Part model, mm, in its own coordinate system. A direction names the side the tool comes from. Round coordinates to 2 decimals unless told otherwise and drop trailing zeros. Write each loop counter-clockwise with the first axis right and the second up, starting at its lowest first coordinate (ties: lowest second). Pieces come first, ordered by that corner, then holes.
1) Flat gauge pins, fed straight in: pin 1 (12 mm diameter, centred on y = 2, z = 15, fed in from -X); pin 2 (15 mm diameter, centred on y = -8.5, z = -2, fed in from +X); pin 3 (21 mm diameter, centred on y = 9, z = -3, fed in from -X). Where does each tip first touch, or does it go through?
2) Drill centre lines: L1, parallel to X at y = 24, z = -9.5; L2, parallel to Z at x = 51, y = -9.5 (3 decimals); L3, parallel to Z at x = -148, y = -8 (3 decimals). Where is each one in solid material? Low to high.
3) Which spindle directions (+Z, -Z, +X, -X, +Y, -Y) get a long thin tool onto all of the face, cutting with end or side? Do faces 1 (the cylindrical face through (116.458, -0.533, 13.965)), 2 (the flat face through (127.794, -1, 0)), 3 (the flat face through (-14, -38.1, 17)). Say none if no direction does.
4) Saw through at B-B on z = -19. Write the cut outline in (x, y) (1 decimal), and give its area (3 significant figures).
5) Saw through at D-D on y = 0. Count the separate pieces of the cut face and the enclosed holes in it, and give its area (3 significant figures).
6) Saw through at A-A on z = 5. Write the cut outline in (x, y), and give its area (3 significant figures).
7) Pull direction X, two halves, no side cores. Call faces 4 (the cylindrical face through (123.02, -0.533, 20.873)), 5 (the flat face through (118.269, -1, 0)), 6 (the flat face through (-14, 38.1, 17)): +X half, -X half, draft (parallel to the pull), parting line (faces both ways), or undercut.
8) Saw through at C-C on y = 29. Write the cut outline in (x, z) (3 decimals), and give its area (3 significant figures).
```python
from build123d import *

# Parameters (mm, degrees)
F1_DEPTH = 38.1
F2_R     = 6.35
F3_R     = 15.875
F4_R     = 8.73125
F5_DEPTH = 25.4
F6_R     = 7.14375
F7_DEPTH = 25.4


with BuildPart() as f1:
    # F0 (on Front) → F1 (new body, symmetric)
    with BuildSketch(Plane.XZ):
        Polygon((-178.59375, -15.875), (-178.59375, -25.4), (-118.26875, -25.4), (-118.26875, 15.875), (118.26875, 15.875), (118.26875, -25.4), (178.59375, -25.4), (178.59375, -15.875), (127.79375, -15.875), (127.79375, 25.4), (-127.79375, 25.4), (-127.79375, -15.875), align=None)
    extrude(amount=F1_DEPTH, both=True)

    # F2
    f2_edges = [f1.edges().sort_by_distance(p)[0] for p in [
        (-127.79375, 0, -15.875),
        (-118.26875, 0, 15.875),
        (118.26875, 0, 15.875),
        (127.79375, 0, -15.875),
    ]]
    fillet(f2_edges, radius=F2_R)

    # F3
    f3_edges = [f1.edges().sort_by_distance(p)[0] for p in [
        (-127.79375, 0, 25.4),
        (127.79375, 0, 25.4),
        (118.26875, 0, -25.4),
        (-118.26875, 0, -25.4),
    ]]
    fillet(f3_edges, radius=F3_R)

    # F4 (on face) → F5 (cut)
    with BuildSketch(Plane.XY.offset(25.4)):
        with Locations((-96.8375, 0)):
            Circle(F4_R)
        with Locations((96.8375, 0)):
            Circle(F4_R)
    extrude(amount=-F5_DEPTH, mode=Mode.SUBTRACT)

    # F6 (on face) → F7 (cut)
    with BuildSketch(Plane.XY.offset(-15.875)):
        with Locations((-154.78125, 0)):
            Circle(F6_R)
        with Locations((154.78125, 0)):
            Circle(F6_R)
    extrude(amount=-F7_DEPTH, mode=Mode.SUBTRACT)


solid = f1.part
```
Completed:
1. pin 1: stops at x = -127.79
1. pin 2: stops at x = 127.79
1. pin 3: stops at x = -129.19
2. L1: x = -127.79 to -118.27, 118.27 to 127.79
2. L2: z = 15.875 to 25.4
2. L3: z = -25.4 to -15.875
3. face 1: -Z, +Y, -Y
3. face 2: +Z, +X, +Y, -Y
3. face 3: +Z, -Z, +X, -X, -Y
4. outline: (-178.6, -38.1) - (-121.4, -38.1) - (-121.4, 38.1) - (-178.6, 38.1) - close; (121.4, -38.1) - (178.6, -38.1) - (178.6, 38.1) - (121.4, 38.1) - close; hole circle Ø14.3 at (-154.8, 0); hole circle Ø14.3 at (154.8, 0)
4. area: 8,390 mm2
5. separate pieces: 5
5. enclosed holes: 0
5. area: 3,400 mm2
6. outline: (-127.79, -38.1) - (-118.27, -38.1) - (-118.27, 38.1) - (-127.79, 38.1) - close; (118.27, -38.1) - (127.79, -38.1) - (127.79, 38.1) - (118.27, 38.1) - close
6. area: 1,450 mm2
7. face 4: +X half
7. face 5: undercut
7. face 6: draft
8. outline: (-178.594, -25.4) - (-134.144, -25.4) arc R15.875 ccw to (-118.269, -9.525) - (-118.269, 9.525) arc R6.35 cw to (-111.919, 15.875) - (111.919, 15.875) arc R6.35 cw to (118.269, 9.525) - (118.269, -9.525) arc R15.875 ccw to (134.144, -25.4) - (178.594, -25.4) - (178.594, -15.875) - (134.144, -15.875) arc R6.35 cw to (127.794, -9.525) - (127.794, 9.525) arc R15.875 ccw to (111.919, 25.4) - (-111.919, 25.4) arc R15.875 ccw to (-127.794, 9.525) - (-127.794, -9.525) arc R6.35 cw to (-134.144, -15.875) - (-178.594, -15.875) - close
8. area: 4,010 mm2
